Verification items for the finished model (mm, model axes). A direction names the side the tool comes from. Round coordinates to 2 decimals unless told otherwise and drop trailing zeros. Order: outer loops, then holes, each group sorted by start corner. A loop starts at its lowest first (then second) coordinate and runs counter-clockwise, first axis right, second up. Notation, with made-up numbers: (18.5, 49) -> (25.5, 49) arc R20 cw to (25.5, 54) -> close; hole circle Ø7 at (89, 61.25). An arc over 180 degrees is marked (long way). Return JSON: item names as keys, results as strings. Group by question number.
Item 1: Access from +Z, -Z, +X, -X, +Y, -Y to the whole of each face (thin tool, end or side, straight path). Record for faces 1 (the cylindrical face through (11.923, -3.755, 0.493)), 2 (the flat face through (-8, -10, 1)).
Item 2: Scan lines: probe 1 along Y at (x, z) = (0, 2.1); probe 2 along Y at (x, z) = (0, 0.25); probe 3 along X at (y, z) = (-7, 3.75). Record each from-to range of solid material in increasing order. Write a range as from..to.
Item 3: Sectioned sample at C-C on z = 3.6. Record the cut outline in (x, y).
Item 4: Sectioned sample at A-A on y = 0. Record the cut outline in (x, z).
Item 5: Depth check by flat-ended pin: pin 1 Ø3 at (x, y) = (-7, -13.5) entering from -Z; pin 2 Ø15 at (x, y) = (-1, 0) entering from +Z; pin 3 Ø2 at (x, z) = (2, 4.5) entering from -Y; pin 4 Ø2 at (x, z) = (-5.5, 3) entering from +Y. Enter the tip coordinate at first touch or a pass-through.
Item 6: Draft check along Y on faces 3 (the cylindrical face through (-11.78, 9.04, 2.73)), 4 (the cylindrical face through (-4.01, 18.06, 2.73)), 5 (the flat face through (13.25, 8.08, 5)). Enter one of: pulls with the +Y half, pulls with the -Y half, needs draft (parallel to the pull), parting line crosses it, or undercut.
Autodesk Inventor part; units mm, degrees
ref_plane "YZ Plane" through (0, 0, 0) normal (1, 0, 0) x (0, 1, 0)
ref_plane "XZ Plane" through (0, 0, 0) normal (0, 1, 0) x (-1, 0, 0)
ref_plane "XY Plane" through (0, 0, 0) normal (0, 0, 1) x (1, 0, 0)
sketch "Sketch1" plane through (0, 0, 0) normal (0, 0, 1) x (1, 0, 0)
  circle A0 centre (0, 0) radius 14.85
  circle A1 centre (0, 0) radius 18.5
  circle A2 centre (0, 0) radius 19.25
  circle A3 centre (0, 0) radius 12.5
  dimension "d0" = 29.7
  dimension "d1" = 37
  dimension "d2" = 38.5
  dimension "d8" = 25
extrude "Extrusion1" add sketch "Sketch1" along normal blind 5 contours A1
extrude "Extrusion2" add sketch "Sketch1" along normal blind 1
fillet "Fillet1" radius 0.5 2 edges at (-14.85, 0, 5) (-18.5, 0, 5)
properties part number "Mitutoyo-BD-black-ring"
Recorded:
{
 "1": {"face 1": "+Z, -Z", "face 2": "+Z"},
 "2": {"probe 1": "-18.5..-14.85, 14.85..18.5", "probe 2": "-19.25..-12.5, 12.5..19.25", "probe 3": "-17.12..-13.1, 13.1..17.12"},
 "3": {"outline": "circle Ø37 at (0, 0); hole circle Ø29.7 at (0, 0)"},
 "4": {"outline": "(-19.25, 0) -> (-12.5, 0) -> (-12.5, 1) -> (-14.85, 1) -> (-14.85, 4.5) arc R0.5 ccw to (-15.35, 5) -> (-18, 5) arc R0.5 ccw to (-18.5, 4.5) -> (-18.5, 1) -> (-19.25, 1) -> close; (12.5, 0) -> (19.25, 0) -> (19.25, 1) -> (18.5, 1) -> (18.5, 4.5) arc R0.5 ccw to (18, 5) -> (15.35, 5) arc R0.5 ccw to (14.85, 4.5) -> (14.85, 1) -> (12.5, 1) -> close"},
 "5": {"pin 1": "z = 0", "pin 2": "through", "pin 3": "y = -18.47", "pin 4": "y = 17.94"},
 "6": {"face 3": "undercut", "face 4": "parting line crosses it", "face 5": "needs draft"}
}
